from build123d import *

# Parameters (mm, degrees)
BOSS_EXTRUDE1_DEPTH   = 22.5
M4X0_7_TAPPED_HOLE2_D = 3.3
REVOLVE1_ANGLE        = 180
BOSS_EXTRUDE4_REACH   = 42.5
M3X0_5_TAPPED_HOLE1_D = 2.5
SKETCH2_R             = 3
CUT_EXTRUDE1_DEPTH    = 50
CUT_EXTRUDE3_START    = -10
CUT_EXTRUDE3_DEPTH    = 4


with BuildPart() as part:
    # Sketch1 → Boss-Extrude1 (new body, symmetric)
    with BuildSketch(Plane.XY):
        with BuildLine():
            Line((-15, 7.5), (-15, 9.5))
            Line((-15, 9.5), (15, 9.5))
            Line((15, 9.5), (15, 7.5))
            ThreePointArc((15, 7.5), (7.5, 0), (15, -7.5))
            Line((15, -7.5), (15, -10))
            Line((15, -10), (-15, -10))
            Line((-15, -10), (-15, -7.5))
            ThreePointArc((-15, -7.5), (-7.5, 0), (-15, 7.5))
        make_face()
    extrude(amount=BOSS_EXTRUDE1_DEPTH, both=True)

    # M4x0.7 Tapped Hole2 (through all)
    with Locations(Plane(origin=(0, -10, 0), x_dir=(-1, 0, 0), z_dir=(0, -1, 0))):
        with Locations((0, -17.5), (0, 17.5)):
            Hole(M4X0_7_TAPPED_HOLE2_D / 2)

    # Sketch12 → Revolve1 (revolve, symmetric)
    with BuildSketch(Plane.XY) as revolve1_sk:
        Polygon((8, -31), (8, -24.5), (6, -24.5), (6, -19), (8, -19), (8, -10), (15, -10), (15, -31), align=None)
    revolve(axis=Axis((0, 0, 0), (0, -1, 0)), revolution_arc=REVOLVE1_ANGLE / 2)
    revolve(revolve1_sk.sketch, axis=Axis((0, 0, 0), (0, 1, 0)), revolution_arc=REVOLVE1_ANGLE / 2)

    # Sketch15 → Boss-Extrude4 (add, up to next)
    with BuildSketch(Plane.XZ.offset(31), mode=Mode.PRIVATE) as boss_extrude4_sk1:
        with BuildLine():
            Line((15, 15), (0, 15))
            ThreePointArc((0, 15), (10.606601729, 10.606601707), (15, -3.1e-08))
            Line((15, -3.1e-08), (15, 15))
        make_face()
    boss_extrude4_tool1 = extrude(boss_extrude4_sk1.sketch, amount=-BOSS_EXTRUDE4_REACH, mode=Mode.PRIVATE) - part.part
    add(boss_extrude4_tool1.solids().sort_by_distance((11.649481, -31, 11.649481))[0])
    # Sketch15 → Boss-Extrude4 (add, up to next)
    with BuildSketch(Plane.XZ.offset(31), mode=Mode.PRIVATE) as boss_extrude4_sk2:
        with BuildLine():
            Line((15, -15), (15, -3.1e-08))
            ThreePointArc((15, -3.1e-08), (10.606601707, -10.606601729), (0, -15))
            Line((0, -15), (15, -15))
        make_face()
    boss_extrude4_tool2 = extrude(boss_extrude4_sk2.sketch, amount=-BOSS_EXTRUDE4_REACH, mode=Mode.PRIVATE) - part.part
    add(boss_extrude4_tool2.solids().sort_by_distance((11.649481, -31, -11.649481))[0])

    # M3x0.5 Tapped Hole1 (through all)
    with Locations(Plane.ZY):
        with Locations((-11.5, -17.75), (-11.5, -25.75), (11.5, -25.75), (11.5, -17.75)):
            Hole(M3X0_5_TAPPED_HOLE1_D / 2)

    # Sketch2 → Cut-Extrude1 (cut)
    with BuildSketch(Plane(origin=(0, 9.5, 0), x_dir=(1, 0, 0), z_dir=(0, 1, 0))):
        Circle(SKETCH2_R)
    extrude(amount=-CUT_EXTRUDE1_DEPTH, mode=Mode.SUBTRACT)

    # Sketch11 → Cut-Extrude3 (cut)
    with BuildSketch(Plane(origin=(0, 0, -22.5), x_dir=(-1, 0, 0), z_dir=(0, 0, -1)).offset(CUT_EXTRUDE3_START)):
        with BuildLine():
            Line((-5, 9.5), (-5, 0))
            ThreePointArc((-5, 0), (-7.928932188, -7.071067812), (-15, -10))
            Line((-15, -10), (-15, -12))
            Line((-15, -12), (-3.5, -12))
            Line((-3.5, -12), (-3.5, -10))
            Line((-3.5, -10), (-3.5, 9.5))
            Line((-3.5, 9.5), (-5, 9.5))
        make_face()
        with BuildLine():
            Line((3.5, 9.5), (5, 9.5))
            Line((5, 9.5), (5, 0))
            ThreePointArc((5, 0), (7.928932188, -7.071067812), (15, -10))
            Line((15, -10), (15, -12))
            Line((15, -12), (3.5, -12))
            Line((3.5, -12), (3.5, -10))
            Line((3.5, -10), (3.5, 9.5))
        make_face()
    cut_extrude3 = extrude(amount=-CUT_EXTRUDE3_DEPTH, mode=Mode.SUBTRACT)

    # Mirror1: Cut-Extrude3 across plane
    add(cut_extrude3.mirror(Plane.XY), mode=Mode.SUBTRACT)


solid = part.part
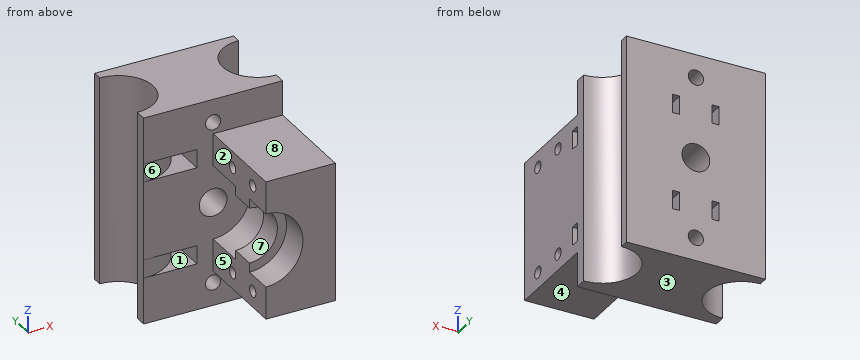
Geometry check sheet. Reference: the model listing, model coordinates, mm. Face numbers are marked on the shaded views. A direction names the side the tool comes from. Coordinates: 2 decimals unless noted, no trailing zeros. Order: outer loops, then holes, each group sorted by start corner. A loop starts at its lowest first (then second) coordinate and runs counter-clockwise, first axis right, second up. Notation, with made-up numbers: (-11, 56.25) - (16, 56.25) arc R19 ccw to (16, 70.25) - close; hole circle Ø3 at (29, 22.5). An arc over 180 degrees is marked (long way). One line per item, written item: value.
(1) Sectioned sample at A-A (z = 0). Enter the section's corners in (x, y).
Data:
outline: (-15, -10) - (-3, -10) - (-3, 9.5) - (-15, 9.5) - (-15, 7.5) arc R7.5 cw to (-15, -7.5) - close; (3, -10) - (8, -10) - (8, -19) - (6, -19) - (6, -24.5) - (8, -24.5) - (8, -31) - (15, -31) - (15, -7.5) arc R7.5 cw to (15, 7.5) - (15, 9.5) - (3, 9.5) - close
(2) Access from +Z, -Z, +X, -X, +Y, -Y to the whole of each face (thin tool, end or side, straight path). Record for the marked faces 4, 5, 6, 7 and 8.
Data:
face 4: -Z, +X, -X, -Y
face 5: +Z, -Z, -X, -Y
face 6: -Y
face 7: -X, -Y
face 8: +Z, +X, -X, -Y
(3) Release check for a two-part mould opening along X. For the marked faces 1, 2 and 3 record: +X half, -X half, draft (parallel to the pull), parting line (faces both ways), or undercut.
Data:
face 1: undercut
face 2: -X half
face 3: draft
(4) Thickness scan on probe 1 along Y at (x, z) = (4.75, -11.5); probe 2 along Z at (x, y) = (0, 4.5); probe 3 along X at (y, z) = (4, -9.5). Record the ranges inside material, lowest first. Write a range as from..to.
Data:
probe 1: y = -31..-27, -24.5..-19, -16.5..-12
probe 2: z = -22.5..-19.15, -15.85..-3, 3..15.85, 19.15..22.5
probe 3: x = -8.66..-5, -3.5..3.5, 5..8.66
(5) Depth check by flat-ended pin: pin 1 Ø3 at (x, y) = (4, -20) entering from +Z; pin 2 Ø8 at (y, z) = (1, 6) entering from +X; pin 3 Ø2 at (y, z) = (-25.75, 11.5) entering from +X; pin 4 Ø1.2 at (y, z) = (6, 11.5) entering from -X. Enter the tip coordinate at first touch or a pass-through.
Data:
pin 1: stops at z = 15
pin 2: stops at x = 9.41
pin 3: passes through
pin 4: stops at x = -11.44
(6) Sectioned sample at B-B (y = -17.75). Enter the section's corners in (x, z).
Data:
outline: (0, -15) - (15, -15) - (15, -12.75) - (0, -12.75) - close; (0, -10.25) - (15, -10.25) - (15, 10.25) - (0, 10.25) - (0, 8) arc R8 cw to (0, -8) - close; (0, 12.75) - (15, 12.75) - (15, 15) - (0, 15) - close
(7) Sectioned sample at D-D (z = 11.5). Enter the section's corners in (x, y).
Data:
outline: (-15, -10) arc R10 ccw to (-5, 0) - (-5, 9.5) - (-15, 9.5) - (-15, 7.5) arc R7.5 cw to (-15, -7.5) - close; (-3.5, -10) - (0, -10) - (0, -16.5) - (15, -16.5) - (15, -12) - (3.5, -12) - (3.5, 9.5) - (-3.5, 9.5) - close; (0, -31) - (15, -31) - (15, -27) - (0, -27) - close; (0, -24.5) - (15, -24.5) - (15, -19) - (0, -19) - close; (5, 0) arc R10 ccw to (15, -10) - (15, -7.5) arc R7.5 cw to (15, 7.5) - (15, 9.5) - (5, 9.5) - close
(8) Sectioned sample at C-C (x = -10.5). Enter the section's corners in (y, z), and give its area (3 significant figures).
Data:
outline: (-10, -22.5) - (-6, -22.5) - (-6, 22.5) - (-10, 22.5) - (-10, 12.5) - (-8.93, 12.5) - (-8.93, 8.5) - (-10, 8.5) - (-10, -8.5) - (-8.93, -8.5) - (-8.93, -12.5) - (-10, -12.5) - close; (6, -22.5) - (9.5, -22.5) - (9.5, 22.5) - (6, 22.5) - close
area: 329 mm^2
